Build history of the part. All positions in model axes, mm. Face numbers are marked on the shaded views. A direction names the side the tool comes from. Round coordinates to 2 decimals unless told otherwise and drop trailing zeros. Write each loop counter-clockwise with the first axis right and the second up, starting at its lowest first coordinate (ties: lowest second). Pieces come first, ordered by that corner, then holes.
Autodesk Inventor part; units mm, degrees
ref_plane "YZ Plane" through (0, 0, 0) normal (1, 0, 0) x (0, 1, 0)
ref_plane "XZ Plane" through (0, 0, 0) normal (0, 1, 0) x (-1, 0, 0)
ref_plane "XY Plane" through (0, 0, 0) normal (0, 0, 1) x (1, 0, 0)
sketch "Sketch1" plane through (0, 0, 0) normal (0, 1, 0) x (-1, 0, 0)
  line L0 (-3.5, 15.724) -> (3.5, 15.724)
  line L1 (3.5, 15.724) -> (3.5, -15.724)
  line L2 (3.5, -15.724) -> (-3.5, -15.724)
  line L3 (-3.5, -15.724) -> (-3.5, 15.724)
  line L4 (-3.5, 15.724) -> (3.5, -15.724) construction
  line L5 (3.5, 15.724) -> (-3.5, -15.724) construction
  line L6 (3.5, 15.724) -> (3.5, 11.724)
  point P0 (0, 0)
  dimension "d0" = 7
  dimension "d1" = 4
extrude "Extrusion1" add sketch "Sketch1" along normal blind 7
sketch "Sketch2" plane through (-3.5, 0, -15.724) normal (-1, 0, 0) x (0, 0, 1)
  line L0 (31.4479, 7) -> (0, 7)
  line L1 (31.4479, 7) -> (27.4406, 7)
  line L2 (0, 7) -> (4.5, 7)
  line L3 (4.5, 7) -> (4.5, 2.0159)
  line L4 (4.5, 2.0159) -> (0, 2.0159)
  line L5 (0, 2.0159) -> (0, 7)
  line L6 (27.4406, 7) -> (24.383, 7)
  line L7 (24.383, 7) -> (24.383, 2.0159)
  line L8 (24.383, 2.0159) -> (27.4406, 2.0159)
  line L9 (27.4406, 2.0159) -> (27.4406, 7)
  point P0 (15.724, 0)
  point P1 (4.5, 7)
  dimension "d4" = 4.5
extrude "Extrusion2" add sketch "Sketch2" along normal blind 30
properties part number "JoystickHållare"
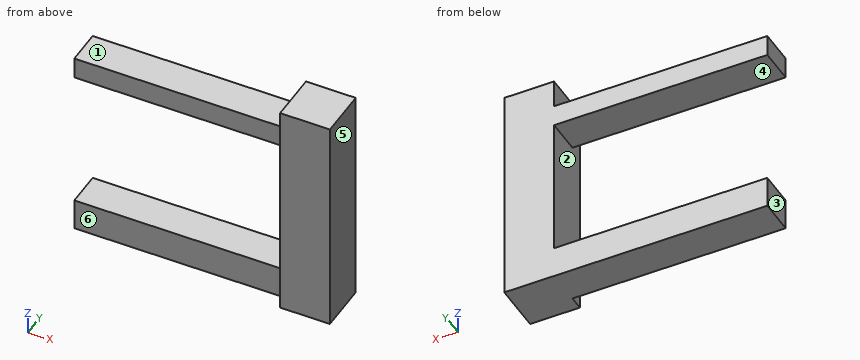
1) Slice it at D-D (y = 1). Write the cut outline in (x, z).
Results:
outline: (-3.5, -15.72) - (3.5, -15.72) - (3.5, 15.72) - (-3.5, 15.72) - close
2) Slice it at B-B (z = 9.5). Write the cut outline in (x, y), plus the area to 3 significant figures.
Results:
outline: (-33.5, 2.02) - (-3.5, 2.02) - (-3.5, 0) - (3.5, 0) - (3.5, 7) - (-33.5, 7) - close
area: 199 mm2
3) Mould opens along Z. For the marked faces 1, 2 and 3 say: released by +Z, released by -Z, zero draft, split by the parting line, or undercut.
Results:
face 1: released by +Z
face 2: undercut
face 3: zero draft
4) Which spindle directions (+Z, -Z, +X, -X, +Y, -Y) get a long thin tool onto all of the face, cutting with end or side? Do the marked faces 4, 5 and 6. Say none if no direction does.
Results:
face 4: -X, +Y, -Y
face 5: +Z, -Z, +X, +Y, -Y
face 6: +Z, -Z, -X, -Y
5) Pin check, flat tips, straight feed: pin 1 Ø1.5 at (x, y) = (-8.5, 3) entering from +Z; pin 2 Ø0.9 at (x, z) = (-18, 10) entering from -Y; pin 3 Ø2 at (y, z) = (2, 1.5) entering from -X. Stop position of each tip, or through.
Results:
pin 1: stops at z = 11.72
pin 2: stops at y = 2.02
pin 3: stops at x = -3.5
6) Slice it at C-C (y = 4.5). Write the cut outline in (x, z).
Results:
outline: (-33.5, -15.72) - (3.5, -15.72) - (3.5, 15.72) - (-3.5, 15.72) - (-3.5, 11.72) - (-33.5, 11.72) - (-33.5, 8.66) - (-3.5, 8.66) - (-3.5, -11.22) - (-33.5, -11.22) - close
7) Wall check: L1, parallel to Z at x = -6, y = 4; L2, parallel to X at y = 0.75, z = -1.5; L3, parallel to Y at x = -13.5, z = 9. Give the ranges that are in metal, low to high.
Results:
L1: z = -15.72 to -11.22, 8.66 to 11.72
L2: x = -3.5 to 3.5
L3: y = 2.02 to 7
8) Slice it at A-A (x = -4). Write the cut outline in (y, z).
Results:
outline: (2.02, -15.72) - (7, -15.72) - (7, -11.22) - (2.02, -11.22) - close; (2.02, 8.66) - (7, 8.66) - (7, 11.72) - (2.02, 11.72) - close
